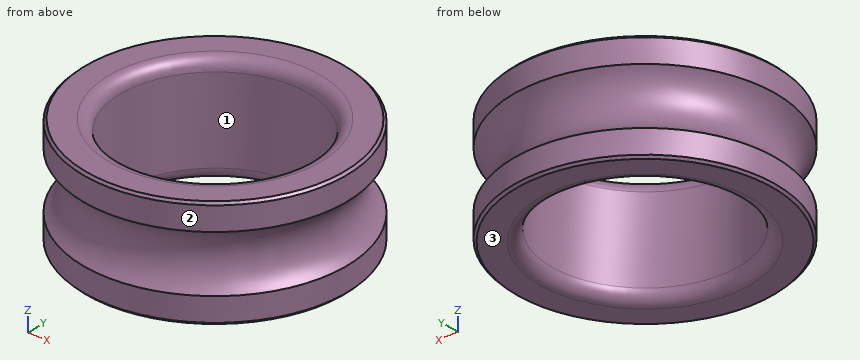
from build123d import *

# Parameters (mm, degrees)
SKETCH1_R           = 28
SKETCH1_R_2         = 20
BOSS_EXTRUDE1_DEPTH = 11.5
SKETCH3_R           = 7.5
CHAMFER1_SIZE       = 0.5
FILLET1_R           = 2.5


with BuildPart() as part:
    # Sketch1 → Boss-Extrude1 (new, symmetric)
    with BuildSketch(Plane.XY):
        Circle(SKETCH1_R)
        Circle(SKETCH1_R_2, mode=Mode.SUBTRACT)
    extrude(amount=BOSS_EXTRUDE1_DEPTH, both=True)

    # Sketch3 → Cut-Revolve1 (revolve, cut)
    with BuildSketch(Plane(origin=(0, 0, 0), x_dir=(1, 0, 0), z_dir=(0, 1, 0))):
        with Locations((32.5, 0)):
            Circle(SKETCH3_R)
    revolve(axis=Axis((0, 0, 0), (0, 0, -1)), mode=Mode.SUBTRACT)

    # Chamfer1
    chamfer1_edges = [part.edges().sort_by_distance(p)[0] for p in [
        (-28, 0, -11.5),
        (-28, 0, 11.5),
    ]]
    chamfer(chamfer1_edges, length=CHAMFER1_SIZE)

    # Fillet1
    fillet1_edges = [part.edges().sort_by_distance(p)[0] for p in [
        (-20, 0, -11.5),
        (-20, 0, 11.5),
    ]]
    fillet(fillet1_edges, radius=FILLET1_R)


solid = part.part
Design review of the part built by this model. Coordinates are the model's own, in mm. Face numbers are marked on the shaded views. Give positions to 0.01 mm unless a question says otherwise; leave off trailing zeros. Write each loop counter-clockwise with the first axis right and the second up, starting at its lowest first coordinate (ties: lowest second). Pieces come first, ordered by that corner, then holes. Notation, with made-up numbers: M -27,-35 L 0,-35 A26 ccw 0,-10 Z; hole C 9,43.25 d7. An arc over 180 degrees is marked long. Answer as a JSON object with one key per item and string values. Group by question number.
1) We need section C-C (z = -4.5). Give the boundary of the cut face in (x, y).
2) For line 1 along Y through (x, z) = (0, 3.75); line 2 along X through (y, z) = (-4.5, -3); line 3 along Y through (x, z) = (14, 3), list the stretches that pass through material, from the lowest coordinate up.
3) We need section D-D (z = 2). Give the boundary of the cut face in (x, y).
4) We need section A-A (y = 0). Give the boundary of the cut face in (x, z).
5) Mouldability with a two-part tool opening along Y and no side actions: class the marked faces 1, 2 and 3 as released by +Y, released by -Y, zero draft, split by the parting line, or undercut.
6) Clearance check with flat-ended pins moving along their axes: pin 1 Ø12 at (x, y) = (1, -15) entering from -Z; pin 2 Ø12 at (y, z) = (10.5, -5) entering from +X; pin 3 Ø8 at (y, z) = (13.5, -1.5) entering from -X. State where each tip first meets the part, or that it passes through.
Answer key:
{
 "1": {"outline": "C 0,0 d53; hole C 0,0 d40"},
 "2": {"line 1": "y = -26 to -20, 20 to 26", "line 2": "x = -25.23 to -19.49, 19.49 to 25.23", "line 3": "y = -21.46 to -14.28, 14.28 to 21.46"},
 "3": {"outline": "C 0,0 d50.54; hole C 0,0 d40"},
 "4": {"outline": "M -28,-11 L -27.5,-11.5 L -22.5,-11.5 A2.5 ccw -20,-9 L -20,9 A2.5 ccw -22.5,11.5 L -27.5,11.5 L -28,11 L -28,6 A7.5 cw -28,-6 Z; M 20,-9 A2.5 ccw 22.5,-11.5 L 27.5,-11.5 L 28,-11 L 28,-6 A7.5 cw 28,6 L 28,11 L 27.5,11.5 L 22.5,11.5 A2.5 ccw 20,9 Z"},
 "5": {"face 1": "undercut", "face 2": "split by the parting line", "face 3": "zero draft"},
 "6": {"pin 1": "stops at z = -11.02", "pin 2": "stops at x = 27.62", "pin 3": "stops at x = -24.31"}
}
